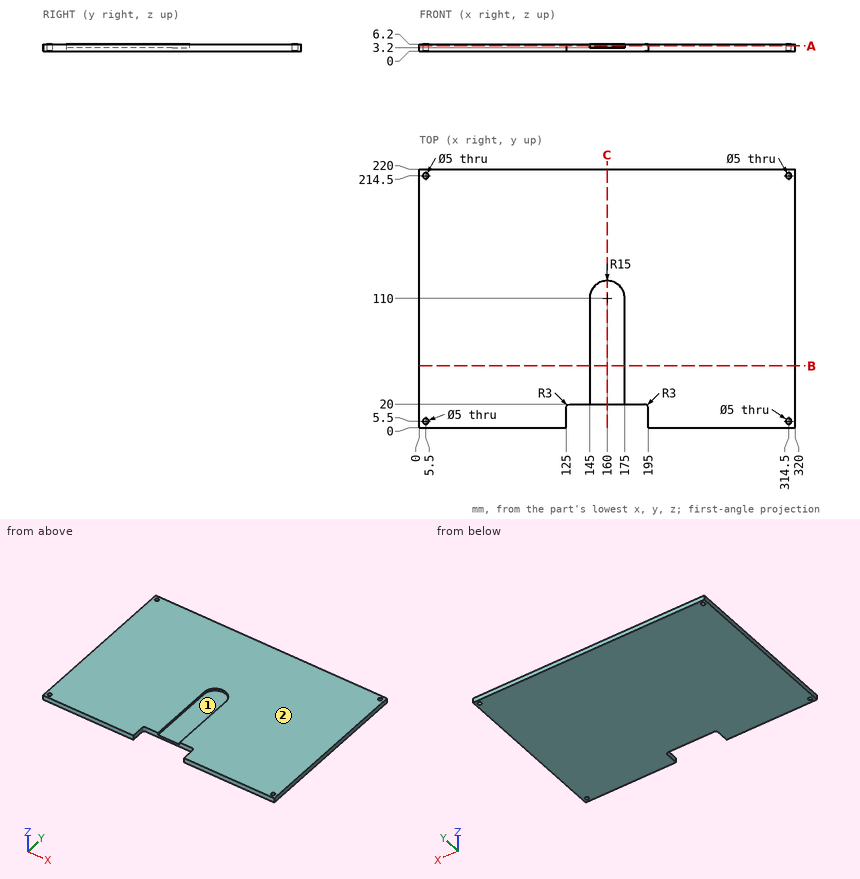
Part print with two shaded views. Sizes in mm from the minimum x, y, z corner. Coordinates: 2 decimals unless noted, no trailing zeros. Loops run counter-clockwise (first coordinate to the right, second up) from the corner with the lowest first, then second, coordinate; pieces in that order, holes last. Notation, with made-up numbers: M -9,-25.5 L 22,-25.5 A23 cw 22,7.5 Z; hole C -20.75,38 d11. An arc over 180 degrees is marked long. Use CSV: the item, a comma, the result in double quotes. Start each with the question number.
1. Band-saw the part on B-B, the plane y = 52.5. List the corners of the cut face in (x, z).
2. Two-plate mould, pull along X, no slides. Class the marked faces 1 and 2: pulls with the +X half, pulls with the -X half, needs draft (parallel to the pull), parting line crosses it, or undercut.
3. Flat gauge pin, fed straight in: pin 1 (4 mm diameter, centred on x = 314.5, y = 5.5, fed in from -Z). Where does the tip first touch, or does it go through?
4. Band-saw the part on C-C, the plane x = 160. List the corners of the cut face in (y, z).
5. Band-saw the part on A-A, the plane z = 4.5. List the corners of the cut face in (x, y), then the cut area to 3 significant figures.
6. Probe probe 1 along X at (y, z) = (214.5, 3.75); probe 2 along Y at (x, z) = (314.5, 2); probe 3 along X at (y, z) = (74, 4.5). List the from-to ranges inside material, lowest first. Write a range as [from, to].
Entries:
1,outline,"M 0,0 L 320,0 L 320,6.2 L 175,6.2 L 175,3.2 L 145,3.2 L 145,6.2 L 0,6.2 Z"
2,face 1,"undercut"
2,face 2,"needs draft"
3,pin 1,"passes through"
4,outline,"M 20,0 L 220,0 L 220,6.2 L 125,6.2 L 125,3.2 L 20,3.2 Z"
5,outline,"M 0,0 L 125,0 L 125,17 A3 cw 128,20 L 145,20 L 145,110 A15 cw 175,110 L 175,20 L 192,20 A3 cw 195,17 L 195,0 L 320,0 L 320,220 L 0,220 Z; hole C 5.5,5.5 d5; hole C 5.5,214.5 d5; hole C 314.5,5.5 d5; hole C 314.5,214.5 d5"
5,area,"65,900 mm2"
6,probe 1,"x = [0, 3], [8, 312], [317, 320]"
6,probe 2,"y = [0, 3], [8, 212], [217, 220]"
6,probe 3,"x = [0, 145], [175, 320]"
